For this review, use the dimensioned drawing (mm, ordinates from the lowest corner) and the shaded views. Round coordinates to 2 decimals unless told otherwise and drop trailing zeros. Write each loop counter-clockwise with the first axis right and the second up, starting at its lowest first coordinate (ties: lowest second). Pieces come first, ordered by that corner, then holes. Notation, with made-up numbers: M 52,9.5 L 81,9.5 A34 ccw 81,47.5 Z; hole C 4,85 d7. An arc over 180 degrees is marked long. Use CSV: the item, a comma, the result in double quotes.
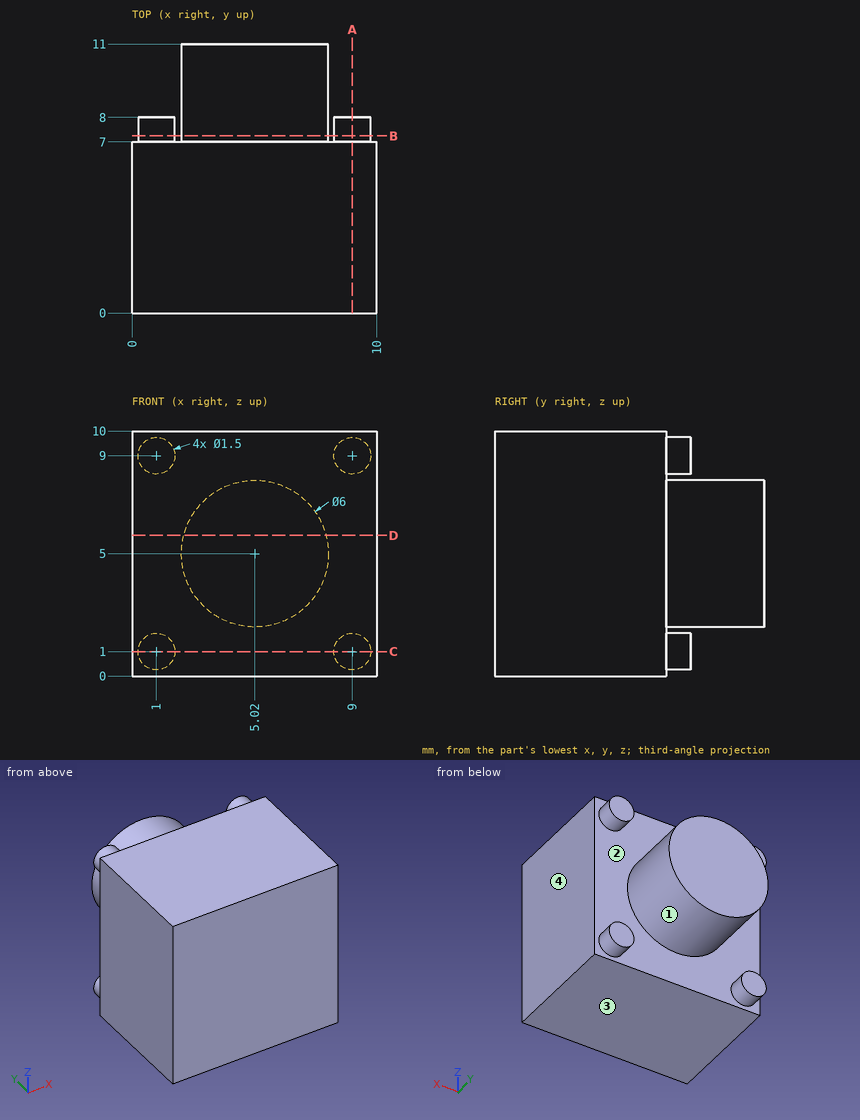
1) The part is to be moulded in two halves that separate along X. For the marked faces 1, 2, 3 and 4, say which applies: released by +X, released by -X, zero draft, split by the parting line, or undercut.
Answers:
face 1,"split by the parting line"
face 2,"undercut"
face 3,"zero draft"
face 4,"released by +X"
2) Add section B-B on y = 7.25. Write out the cut boundary in (x, z).
Answers:
outline,"C 1,1 d1.5; C 1,9 d1.5; C 5.02,5 d6; C 9,1 d1.5; C 9,9 d1.5"
3) Add section A-A on x = 9. Write out the cut boundary in (y, z).
Answers:
outline,"M 0,0 L 7,0 L 7,0.25 L 8,0.25 L 8,1.75 L 7,1.75 L 7,8.25 L 8,8.25 L 8,9.75 L 7,9.75 L 7,10 L 0,10 Z"
4) Wall thickness on line 1 along Z through (x, y) = (9, 7.5); line 2 along Y through (x, z) = (1, 0.75); line 3 along Y through (x, z) = (3.75, 1.5): over which ranges is each line inside the solid? List them lowest first. Write a range as [from, to].
Answers:
line 1,"[0.25, 1.75], [8.25, 9.75]"
line 2,"[0, 8]"
line 3,"[0, 7]"
5) Add section C-C on z = 1. Write out the cut boundary in (x, y).
Answers:
outline,"M 0,0 L 10,0 L 10,7 L 9.75,7 L 9.75,8 L 8.25,8 L 8.25,7 L 1.75,7 L 1.75,8 L 0.25,8 L 0.25,7 L 0,7 Z"
6) For pin 1 Ø2 at (y, z) = (9.5, 6) entering from -X; pin 2 Ø1.6 at (x, z) = (1, 8.5) entering from +Y, all flat-tipped, find the tip position at first contact; note any pin that passes through.
Answers:
pin 1,"x = 2.02"
pin 2,"y = 8"
7) Add section D-D on z = 5.75. Write out the cut boundary in (x, y) (1 decimal).
Answers:
outline,"M 0,0 L 10,0 L 10,7 L 7.9,7 L 7.9,11 L 2.1,11 L 2.1,7 L 0,7 Z"
